Here's the drawing with two shaded views (mm, measured from the low corner). I have some questions. A direction names the side the tool comes from. Coordinates: 2 decimals unless noted, no trailing zeros. Loops run counter-clockwise (first coordinate to the right, second up) from the corner with the lowest first, then second, coordinate; pieces in that order, holes last. Notation, with made-up numbers: (14.5, 49) -> (63.5, 49) arc R13 ccw to (63.5, 54) -> close; hole circle Ø6 at (34, -38). An arc over 180 degrees is marked (long way). Answer as a JSON object with one key per item and string values. Group by question number.
Q1. I want a section at D-D on z = 2.25. Write out the boundary of the cut face in (x, y), then the cut area to 3 significant figures.
Q2. On a 3-axis mill with a long thin cutter (end or side, diameter ignored), from which of +Z, -Z, +X, -X, +Y, -Y can I reach the whole of each face in a straight line? I mean the marked faces 1, 2, 3 and 4. Say none if no direction works.
Q3. I want a section at C-C on y = 8. Write out the boundary of the cut face in (x, z) (1 decimal).
Q4. I'm going to push flat-ended pins straight in: pin 1 (1.5 mm diameter, centred on x = 4, y = 6, fed in from +Z) (1 decimal); pin 2 (2 mm diameter, centred on x = 2.5, y = 10.5, fed in from -Z); pin 3 (0.9 mm diameter, centred on x = 2.5, y = 2.5, fed in from +Z). Where does each tip first touch, or does it pass through?
Q5. I want a section at A-A on z = 9. Write out the boundary of the cut face in (x, y), then the cut area to 3 significant figures.
Q6. I need wall thicknesses on line 1 (Y direction, x = 5, z = 6.25); line 2 (Y direction, x = 2, z = 7); line 3 (Z direction, x = 5.5, y = 4.5) (1 decimal). Which ranges of each line are inside material? Lowest first, please.
Q7. Thinking about a two-plate mould opening in Y: for the marked faces 5, 6 and 7, which applies, released by +Y, released by -Y, zero draft, split by the parting line, or undercut?
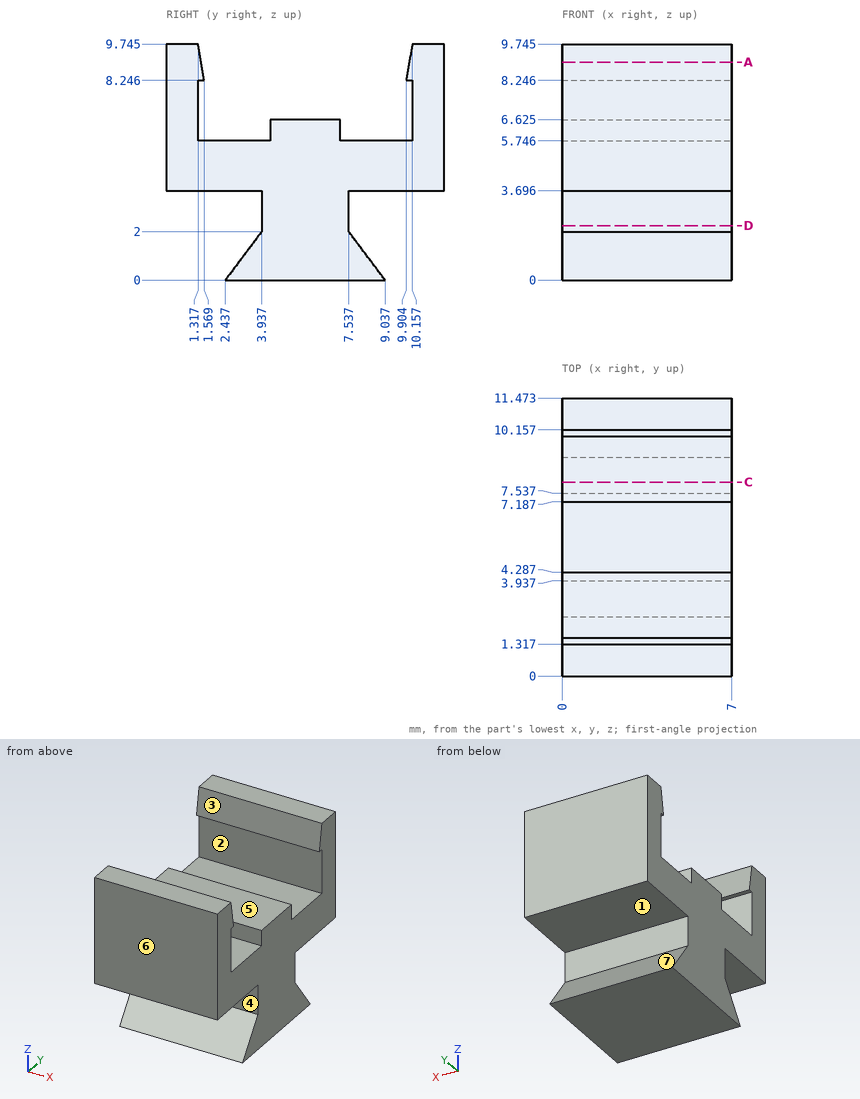
Result set:
{
 "1": {"outline": "(0, 3.94) -> (7, 3.94) -> (7, 7.54) -> (0, 7.54) -> close", "area": "25.2 mm²"},
 "2": {"face 1": "+X, -X, +Y", "face 2": "+X, -X", "face 3": "+Z, +X, -X", "face 4": "+X, -X, -Y"},
 "3": {"outline": "(0, 0) -> (7, 0) -> (7, 1.4) -> (0, 1.4) -> close; (0, 3.7) -> (7, 3.7) -> (7, 5.7) -> (0, 5.7) -> close"},
 "4": {"pin 1": "stops at z = 6.6", "pin 2": "stops at z = 3.7", "pin 3": "stops at z = 5.75"},
 "5": {"outline": "(0, 0) -> (7, 0) -> (7, 1.44) -> (0, 1.44) -> close; (0, 10.03) -> (7, 10.03) -> (7, 11.47) -> (0, 11.47) -> close", "area": "20.2 mm²"},
 "6": {"line 1": "y = 0 to 1.32, 4.29 to 7.19, 10.16 to 11.47", "line 2": "y = 0 to 1.32, 10.16 to 11.47", "line 3": "z = 0 to 6.6"},
 "7": {"face 5": "undercut", "face 6": "released by -Y", "face 7": "released by +Y"}
}
